```python
from build123d import *

# Parameters (mm, degrees)
SKETCH_2_R          = 3.25
CUT_EXTRUDE_1_DEPTH = 3.5


with BuildPart() as part:
    # 草图1 → 旋转1 (revolve)
    with BuildSketch(Plane.XY):
        with BuildLine():
            Line((0, 8), (7, 8))
            Line((7, 8), (7, 4))
            Line((7, 4), (5, 4))
            ThreePointArc((5, 4), (3.585786438, 3.414213562), (3, 2))
            Line((3, 2), (3, -8))
            Line((3, -8), (1.22, -8))
            Line((1.22, -8), (1.22, 0))
            Line((1.22, 0), (0, 0))
            Line((0, 0), (0, 8))
        make_face()
    revolve(axis=Axis((0, -147.558866066, 0), (0, 1, 0)))

    # 草图2 → 切除-拉伸1 (cut, symmetric)
    with BuildSketch(Plane(origin=(0, 0, 0), x_dir=(0, 0, -1), z_dir=(1, 0, 0))):
        with Locations((0, 8)):
            Circle(SKETCH_2_R)
    extrude(amount=CUT_EXTRUDE_1_DEPTH, both=True, mode=Mode.SUBTRACT)


solid = part.part
```
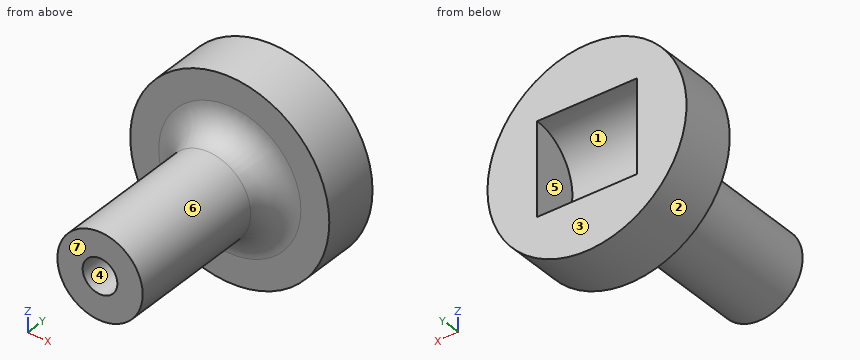
Here's how the part is built. I have some questions about the finished solid (model axes, mm). Face numbers are marked on the shaded views. A direction names the side the tool comes from. Give positions to 0.01 mm unless a question says otherwise; leave off trailing zeros. Loops run counter-clockwise (first coordinate to the right, second up) from the corner with the lowest first, then second, coordinate; pieces in that order, holes last. Notation, with made-up numbers: (84.5, 56) -> (126.5, 56) arc R18 cw to (126.5, 62) -> close; hole circle Ø10 at (-24, 11.25). An arc over 180 degrees is marked (long way). Use one line per item in the form item = value. Start each with the question number.
1) Imagine slicing it at A-A (z = 0). Please give me the cut outline in (x, y).
2) Imagine slicing it at D-D (y = -6.5). Please give me the cut outline in (x, z), then the cut area to 3 significant figures.
3) Imagine slicing it at C-C (y = 1.75). Please give me the cut outline in (x, z).
4) Which directions (+Z, -Z, +X, -X, +Y, -Y) give clear straight access to the entire face, cutting with the end or side of a thin tool? Please do the marked faces 5, 6 and 7.
5) Imagine slicing it at B-B (x = 0). Please give me the cut outline in (y, z), then the cut area to 3 significant figures.
6) For P1, Ø4, axis at x = -5, z = -3, coming from the -Y side; P2, Ø2, axis at x = 0, z = 0, coming from the +Y side; P3, Ø2, axis at y = -6, z = -1, coming from the +X side, each with a flat end and sliding along its axis, tell me the tip position at first contact or that it passes through.
7) Thinking about a two-plate mould opening in Z: for the marked faces 1, 2, 3 and 4, which applies, +Z half, -Z half, draft (parallel to the pull), parting line (faces both ways), or undercut?
8) Please list where these lines run through material, in increasing order: line 1 along X through (y, z) = (-6, 0); line 2 along Y through (x, z) = (-1, 5).
Check values:
q1.outline = (-7, 4) -> (-5, 4) arc R2 cw to (-3, 2) -> (-3, -8) -> (-1.22, -8) -> (-1.22, 0) -> (1.22, 0) -> (1.22, -8) -> (3, -8) -> (3, 2) arc R2 cw to (5, 4) -> (7, 4) -> (7, 8) -> (3.5, 8) -> (3.5, 4.75) -> (-3.5, 4.75) -> (-3.5, 8) -> (-7, 8) -> close
q2.outline = circle Ø6 at (0, 0); hole circle Ø2.44 at (0, 0)
q2.area = 23.6 mm^2
q3.outline = circle Ø6 at (0, 0)
q4.face_5 = +Y
q4.face_6 = -Y
q4.face_7 = +Z, -Z, +X, -X, -Y
q5.outline = (-8, -3) -> (2, -3) arc R2 cw to (4, -5) -> (4, -7) -> (8, -7) -> (8, -3.25) arc R3.25 cw to (8, 3.25) -> (8, 7) -> (4, 7) -> (4, 5) arc R2 cw to (2, 3) -> (-8, 3) -> (-8, 1.22) -> (0, 1.22) -> (0, -1.22) -> (-8, -1.22) -> close
q5.area = 93.6 mm^2
q6.P1 = 3.62
q6.P2 = 4.91
q6.P3 = 3
q7.face_1 = undercut
q7.face_2 = parting line
q7.face_3 = draft
q7.face_4 = undercut
q8.line_1 = -3 to -1.22, 1.22 to 3
q8.line_2 = 4 to 8
